Part model, mm, in its own coordinate system. A direction names the side the tool comes from. Coordinates: 2 decimals unless noted, no trailing zeros. Loops run counter-clockwise (first coordinate to the right, second up) from the corner with the lowest first, then second, coordinate; pieces in that order, holes last. Notation, with made-up numbers: (32.5, 17) -> (52.5, 17) arc R3 cw to (52.5, 22) -> close; hole circle Ø2 at (25, 49.25). An arc over 180 degrees is marked (long way). Use one line per item in the form item = value. Start each with the question number.
(1) Mould opens along X. For faces 1 (the cylindrical face through (20.9, 1.3, 9.7)), 2 (the cylindrical face through (-10, 1.3, -1.8)), 3 (the flat face through (-20, 1, 10)) say: +X half, -X half, draft (parallel to the pull), parting line (faces both ways), or undercut.
(2) 3-axis set-ups, long thin cutter, end or side, ignore diameter. For faces 4 (the flat face through (6, 1, 0)), 5 (the flat face through (-16, 1, 0)), 6 (the flat face through (20, 1, 16)), 7 (the flat face through (-16, 1, 20)): which of +Z, -Z, +X, -X, +Y, -Y reach the whole face in a straight line?
(3) Band-saw the part on B-B on z = 10. Give the cut face in (x, y).
(4) Band-saw the part on D-D on x = 16. Give the cut face in (y, z).
(5) Pin check, flat tip, straight feed: P1, Ø1.3, axis at x = -14.5, y = 0.5, coming from the +Z side. Stop position of the tip, or through.
(6) Band-saw the part on A-A on x = -10. Give the cut face in (y, z), then the cut area to 3 significant figures.
(7) Band-saw the part on C-C on y = 2.15. Give the cut face in (x, z), then the cut area to 3 significant figures.
(8) Drill centre lines: L1, parallel to Z at x = -10, y = 1.75; L2, parallel to X at y = 1.25, z = 10; L3, parallel to X at y = 1.3, z = 16.5. Where is each one in solid material? Low to high. Write a range as [from, to].
```python
from build123d import *

# Parameters (mm, degrees)
SKETCH1_R           = 0.95
BOSS_EXTRUDE1_DEPTH = 2.6


with BuildPart() as part:
    # Sketch1 → Boss-Extrude1 (new body)
    with BuildSketch(Plane(origin=(0, 0, 0), x_dir=(1, 0, 0), z_dir=(0, 1, 0))):
        with BuildLine():
            Line((20, -8.2), (20, 0))
            Line((20, 0), (-8.2, 0))
            ThreePointArc((-8.2, 0), (-10, 1.8), (-11.8, 0))
            Line((-11.8, 0), (-20, 0))
            Line((-20, 0), (-20, -20))
            Line((-20, -20), (-11.8, -20))
            ThreePointArc((-11.8, -20), (-10, -21.8), (-8.2, -20))
            Line((-8.2, -20), (20, -20))
            Line((20, -20), (20, -11.8))
            ThreePointArc((20, -11.8), (21.8, -10), (20, -8.2))
        make_face()
        with Locations((-10, 0)):
            Circle(SKETCH1_R, mode=Mode.SUBTRACT)
        with Locations((20, -10)):
            Circle(SKETCH1_R, mode=Mode.SUBTRACT)
        with Locations((-10, -20)):
            Circle(SKETCH1_R, mode=Mode.SUBTRACT)
    extrude(amount=BOSS_EXTRUDE1_DEPTH)


solid = part.part
```
A:
q1.face_1 = undercut
q1.face_2 = parting line
q1.face_3 = -X half
q2.face_4 = -Z, +X, +Y, -Y
q2.face_5 = -Z, -X, +Y, -Y
q2.face_6 = +Z, +X, +Y, -Y
q2.face_7 = +Z, -X, +Y, -Y
q3.outline = (-20, 0) -> (19.05, 0) -> (19.05, 2.6) -> (-20, 2.6) -> close; (20.95, 0) -> (21.8, 0) -> (21.8, 2.6) -> (20.95, 2.6) -> close
q4.outline = (0, 0) -> (2.6, 0) -> (2.6, 20) -> (0, 20) -> close
q5.P1 = 20
q6.outline = (0, -1.8) -> (2.6, -1.8) -> (2.6, -0.95) -> (0, -0.95) -> close; (0, 0.95) -> (2.6, 0.95) -> (2.6, 19.05) -> (0, 19.05) -> close; (0, 20.95) -> (2.6, 20.95) -> (2.6, 21.8) -> (0, 21.8) -> close
q6.area = 51.5 mm²
q7.outline = (-20, 0) -> (-11.8, 0) arc R1.8 ccw to (-8.2, 0) -> (20, 0) -> (20, 8.2) arc R1.8 ccw to (20, 11.8) -> (20, 20) -> (-8.2, 20) arc R1.8 ccw to (-11.8, 20) -> (-20, 20) -> close; hole circle Ø1.9 at (-10, 0); hole circle Ø1.9 at (-10, 20); hole circle Ø1.9 at (20, 10)
q7.area = 807 mm²
q8.L1 = [-1.8, -0.95], [0.95, 19.05], [20.95, 21.8]
q8.L2 = [-20, 19.05], [20.95, 21.8]
q8.L3 = [-20, 20]
